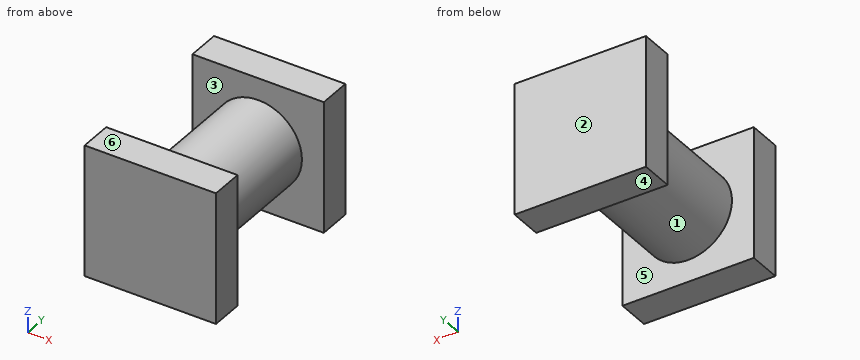
```python
from build123d import *

# Parameters (mm, degrees)
F0_W     = 76.2
F0_H     = 76.2
F1_DEPTH = 19.05
F2_R     = 25.4
F3_DEPTH = 76.2
F4_W     = 78.3899585484
F4_H     = 76.2
F4_R     = 25.4
F5_DEPTH = 19.05
F7_W     = 76.2
F7_H     = 76.2
F7_R     = 25.4
F8_DEPTH = 19.05


with BuildPart() as f1:
    # F0 (on Front) → F1 (new body)
    with BuildSketch(Plane.XZ):
        Rectangle(F0_W, F0_H)
    extrude(amount=F1_DEPTH)

    # F2 (on face) → F3 (join)
    with BuildSketch(Plane.XZ.offset(19.05)):
        Circle(F2_R)
    extrude(amount=F3_DEPTH)

    # F7 (on face) → F8 (join)
    with BuildSketch(Plane.XZ.offset(95.25)):
        Rectangle(F7_W, F7_H)
        Circle(F7_R, mode=Mode.SUBTRACT)
        Circle(F7_R)
    extrude(amount=F8_DEPTH)


with BuildPart() as f5:
    # F4 (on face) → F5 (new body)
    with BuildSketch(Plane.XZ.offset(95.25)):
        Rectangle(F4_W, F4_H)
        Circle(F4_R, mode=Mode.SUBTRACT)
    extrude(amount=F5_DEPTH)


solid = f1.part
```
The model under review builds one solid part; all positions refer to its coordinate system, in mm. Face numbers are marked on the shaded views. A direction names the side the tool comes from. Round coordinates to 2 decimals unless told otherwise and drop trailing zeros. Order: outer loops, then holes, each group sorted by start corner. A loop starts at its lowest first (then second) coordinate and runs counter-clockwise, first axis right, second up.
Item 1: Add section B-B, the plane z = 0. State the section outline as (x, y) points, and give its area (3 significant figures).
Working result:
outline: (-38.1, -114.3) - (38.1, -114.3) - (38.1, -95.25) - (25.4, -95.25) - (25.4, -19.05) - (38.1, -19.05) - (38.1, 0) - (-38.1, 0) - (-38.1, -19.05) - (-25.4, -19.05) - (-25.4, -95.25) - (-38.1, -95.25) - close
area: 6,770 mm2
Item 2: Add section A-A, the plane x = 0. State the section outline as (y, z) points, and give its area (3 significant figures).
Working result:
outline: (-114.3, -38.1) - (-95.25, -38.1) - (-95.25, -25.4) - (-19.05, -25.4) - (-19.05, -38.1) - (0, -38.1) - (0, 38.1) - (-19.05, 38.1) - (-19.05, 25.4) - (-95.25, 25.4) - (-95.25, 38.1) - (-114.3, 38.1) - close
area: 6,770 mm2
Item 3: Add section C-C, the plane y = -70. State the section outline as (x, z) points, and give its area (3 significant figures).
Working result:
outline: circle Ø50.8 at (0, 0)
area: 2,030 mm2
Item 4: Machinability: for the marked faces 5 and 6, which of the approach directions +Z, -Z, +X, -X, +Y, -Y give a long, thin tool a straight path to every point of the face, cutting with its end or side? Answer none if there is none.
Working result:
face 5: none
face 6: +Z, +X, -X, +Y, -Y
Item 5: For pin 1 (10 mm diameter, centred on x = -27, y = -40, fed in from -Z); pin 2 (6 mm diameter, centred on y = -28, z = 25, fed in from -X); pin 3 (1.5 mm diameter, centred on y = -46, z = -15.5, fed in from -X), all flat-tipped, find the tip position at first contact; note any pin that passes through.
Working result:
pin 1: stops at z = -12.69
pin 2: stops at x = -12.69
pin 3: stops at x = -20.68
Item 6: To check wall thickness, follow probe 1 along Y at (x, z) = (-14, -33.5); probe 2 along Z at (x, y) = (-1, -74); probe 3 along Z at (x, y) = (12, -76.5). State the ranges of each line that lie inside material, in increasing order.
Working result:
probe 1: y = -114.3 to -95.25, -19.05 to 0
probe 2: z = -25.38 to 25.38
probe 3: z = -22.39 to 22.39
Item 7: Draft analysis for pull direction Y (two halves, no side actions). For the marked faces 1, 2, 3 and 4, state which applies: released by +Y, released by -Y, zero draft, split by the parting line, or undercut.
Working result:
face 1: undercut
face 2: released by +Y
face 3: undercut
face 4: zero draft
